Geometry check sheet. Reference: the model listing, model coordinates, mm. A direction names the side the tool comes from. Round coordinates to 2 decimals unless told otherwise and drop trailing zeros. Write each loop counter-clockwise with the first axis right and the second up, starting at its lowest first coordinate (ties: lowest second). Pieces come first, ordered by that corner, then holes. Notation, with made-up numbers: (33.25, 8) -> (46.25, 8) arc R32 cw to (46.25, 42) -> close; hole circle Ø10 at (38, 25.25). An arc over 180 degrees is marked (long way). One line per question, with ' | ' between items.
```python
from build123d import *

# Parameters (mm, degrees)
CUT_EXTRUDE_2_DEPTH = 19
CHAMFER_1_SIZE      = 0.8


with BuildPart() as part:
    # Эскиз1 → Повернуть1 (revolve)
    with BuildSketch(Plane(origin=(0, 0, 0), x_dir=(1, 0, 0), z_dir=(0, 1, 0))):
        Polygon((0, 2), (18, 2), (18, 3.175), (8, 3.175), (8, 3.7), (7.7, 4), (2, 4), (2, 7), (0, 7), align=None)
    revolve(axis=Axis((0, 0, 0), (1, 0, 0)))

    # Эскиз2 → Вырез-Вытянуть2 (cut, through all)
    with BuildSketch(Plane.ZY):
        with BuildLine():
            Line((4.898979486, -5), (-4.898979486, -5))
            ThreePointArc((-4.898979486, -5), (0, -7), (4.898979486, -5))
        make_face()
    extrude(amount=-CUT_EXTRUDE_2_DEPTH, mode=Mode.SUBTRACT)

    # Фаска1
    chamfer_1_edges = [part.edges().sort_by_distance(p)[0] for p in [
        (0, 7, 0),
        (2, -5, 0),
    ]]
    chamfer(chamfer_1_edges, length=CHAMFER_1_SIZE)


solid = part.part
```
(1) Material ranges on line 1 (Y direction, x = 7, z = 0); line 2 (Y direction, x = 12.25, z = 0) (3 decimals); line 3 (X direction, y = 4.5, z = -3.5), recorded low to high.
Resolved:
line 1: y = -4 to -2, 2 to 4 | line 2: y = -3.175 to -2, 2 to 3.175 | line 3: x = 0 to 2
(2) Sectioned sample at A-A on z = 0. Record the cut outline in (x, y) (3 decimals).
Resolved:
outline: (0, -5) -> (1.2, -5) -> (2, -4.2) -> (2, -4) -> (7.7, -4) -> (8, -3.7) -> (8, -3.175) -> (18, -3.175) -> (18, -2) -> (0, -2) -> close; (0, 2) -> (18, 2) -> (18, 3.175) -> (8, 3.175) -> (8, 3.7) -> (7.7, 4) -> (2, 4) -> (2, 7) -> (0.8, 7) -> (0, 6.2) -> close
(3) Sectioned sample at C-C on x = 10.25. Record the cut outline in (y, z) (3 decimals).
Resolved:
outline: circle Ø6.35 at (0, 0); hole circle Ø4 at (0, 0)
(4) Sectioned sample at B-B on y = 0. Record the cut outline in (x, z) (3 decimals), then the cut area to 3 significant figures.
Resolved:
outline: (0, -6.2) -> (0.8, -7) -> (2, -7) -> (2, -4) -> (7.7, -4) -> (8, -3.7) -> (8, -3.175) -> (18, -3.175) -> (18, -2) -> (0, -2) -> close; (0, 2) -> (18, 2) -> (18, 3.175) -> (8, 3.175) -> (8, 3.7) -> (7.7, 4) -> (2, 4) -> (2, 7) -> (0.8, 7) -> (0, 6.2) -> close | area: 66.8 mm2
(5) Go/stop test with flat-tipped pins: pin 1 (5 mm diameter, centred on x = 15.5, y = -0.5, fed in from -Z) (3 decimals); pin 2 (3 mm diameter, centred on x = 4.5, y = 2, fed in from -Z). Record where each tip stops, or that it passes through.
Resolved:
pin 1: stops at z = -3.175 | pin 2: stops at z = -3.97
(6) Access from +Z, -Z, +X, -X, +Y, -Y to the whole of each face (thin tool, end or side, straight path). Record for faces 1 (the cylindrical face through (4.81, -3.905, 0.867)), 2 (the flat face through (18, -2, 1)).
Resolved:
face 1: +X | face 2: +Z, -Z, +X, +Y, -Y
(7) Draft check along Z on faces 3 (the flat face through (0, 2, 1)), 4 (the conical face through (0.128, 6.324, 0.222)), 5 (the cylindrical face through (9, -2, 0)). Enter one of: +Z half, -Z half, draft (parallel to the pull), parting line (faces both ways), or undercut.
Resolved:
face 3: draft | face 4: parting line | face 5: undercut
(8) Sectioned sample at D-D on x = 7. Record the cut outline in (y, z), then the cut area to 3 significant figures.
Resolved:
outline: circle Ø8 at (0, 0); hole circle Ø4 at (0, 0) | area: 37.7 mm2
